from build123d import *

# Parameters (mm, degrees)
BOSS_EXTRUDE1_DEPTH = 40.1
SKETCH3_R           = 1.35
CUT_EXTRUDE2_DEPTH  = 50.8
SKETCH4_R           = 1.016
CUT_EXTRUDE3_DEPTH  = 50.8
SKETCH6_W           = 62.086073973
SKETCH6_H           = 34.1
CUT_EXTRUDE4_DEPTH  = 6
BOSS_EXTRUDE5_DEPTH = 2
FILLET1_R           = 1
CUT_EXTRUDE5_DEPTH  = 101.73954578


with BuildPart() as part:
    # Sketch1 → Boss-Extrude1 (new body)
    with BuildSketch(Plane.XY):
        Polygon((0, 0), (0, 52.578), (6, 52.578), (6, 8.5), (76, 8.5), (76, 0), align=None)
    extrude(amount=BOSS_EXTRUDE1_DEPTH)

    # Sketch3 → Cut-Extrude2 (cut)
    with BuildSketch(Plane.XY.offset(40.1)):
        with Locations((27.996, 2.8)):
            Circle(SKETCH3_R)
        with Locations((49.996, 2.8)):
            Circle(SKETCH3_R)
        with Locations((71.996, 2.8)):
            Circle(SKETCH3_R)
    extrude(amount=-CUT_EXTRUDE2_DEPTH, mode=Mode.SUBTRACT)

    # Sketch4 → Cut-Extrude3 (cut)
    with BuildSketch(Plane.ZY):
        with Locations((27.88, 17.6)):
            Circle(SKETCH4_R)
        with Locations(Location((11.88, 17.6, 0), (0, 0, 270))):
            Circle(SKETCH4_R)
        with Locations((27.88, 49.6)):
            Circle(SKETCH4_R)
        with Locations(Location((11.88, 49.6, 0), (0, 0, 270))):
            Circle(SKETCH4_R)
    extrude(amount=-CUT_EXTRUDE3_DEPTH, mode=Mode.SUBTRACT)

    # Sketch6 → Cut-Extrude4 (cut)
    with BuildSketch(Plane.XZ):
        with Locations((50.043036987, 20.05)):
            Rectangle(SKETCH6_W, SKETCH6_H)
    extrude(amount=-CUT_EXTRUDE4_DEPTH, mode=Mode.SUBTRACT)

    # Sketch16 → Boss-Extrude5 (add)
    with BuildSketch(Plane.XY.offset(40.1)):
        Polygon((6, 8.5), (26, 8.5), (6, 33.5), align=None)
    boss_extrude5 = extrude(amount=-BOSS_EXTRUDE5_DEPTH)

    # Mirror2: Boss-Extrude5 across plane
    add(boss_extrude5.mirror(Plane(origin=(0, 0, 20.05), x_dir=(1, 0, 0), z_dir=(0, 0, -1))))

    # Fillet1
    fillet1_edges = [part.edges().sort_by_distance(p)[0] for p in [
        (0, 0, 20.05),
        (76, 0, 38.6),
        (3, 52.578, 40.1),
        (76, 0, 1.5),
        (3, 52.578, 0),
    ]]
    fillet(fillet1_edges, radius=FILLET1_R)

    # Sketch17 → Cut-Extrude5 (cut, through all)
    with BuildSketch(Plane.XY.offset(40.1)):
        with BuildLine():
            Line((17.4625, 0), (17.4625, 8.5))
            Line((17.4625, 8.5), (6, 19.9625))
            Line((6, 19.9625), (6, 33.5))
            Line((6, 33.5), (26, 8.5))
            Line((26, 8.5), (76, 8.5))
            Line((76, 8.5), (76, 1))
            ThreePointArc((76, 1), (75.707106781, 0.292893219), (75, 0))
            Line((75, 0), (17.4625, 0))
        make_face()
    extrude(amount=-CUT_EXTRUDE5_DEPTH, mode=Mode.SUBTRACT)


solid = part.part
The listing builds one solid part. Answer for the finished solid, in the listing's coordinates (mm). A direction names the side the tool comes from. Coordinates: 2 decimals unless noted, no trailing zeros. Loops run counter-clockwise (first coordinate to the right, second up) from the corner with the lowest first, then second, coordinate; pieces in that order, holes last. Notation, with made-up numbers: (-23.75, -4.75) -> (3.25, -4.75) arc R17 ccw to (3.25, 26.25) -> close; hole circle Ø1 at (49, 67). An arc over 180 degrees is marked (long way). Answer in a Markdown table with one row per item. Add a question column.
1. Determine the mould class of faces 1 (the cylindrical face through (2.96, 48.7, 28.35)), 2 (the flat face through (3, 52.578, 20)), 3 (the cylindrical face through (2.958, 18.406, 11.262)), 4 (the flat face through (17.462, 4, 20)) for opening direction Y: +Y half, -Y half, draft (parallel to the pull), parting line (faces both ways), or undercut.
2. The part is cut by section C-C, the plane z = 27.88. Write down the section's boundary in (x, y), then the cut area to 3 significant figures.
3. The part is cut by section D-D, the plane x = 10. Write down the section's boundary in (y, z), then the cut area to 3 significant figures.
4. The part is cut by section A-A, the plane y = 49.6. Write down the section's boundary in (x, z), then the cut area to 3 significant figures.
5. For faces 5 (the flat face through (9, 12, 2)), 6 (the flat face through (5, 20, 0)), determine the directions among +Z, -Z, +X, -X, +Y, -Y from which every point of the face is accessible in a straight line to the end or side of a thin tool.
6. The part is cut by section B-B, the plane z = 23.5. Write down the section's boundary in (x, y), then the cut area to 3 significant figures.
7. Consider line 1 (Y direction, x = 4.8, z = 27.88); line 2 (Y direction, x = 16.25, z = 36); line 3 (X direction, y = 14.5, z = 31). Determine where each line is inside the solid, lowest interval first. Write a range as [from, to].
8. Flat-ended cylindrical pins translate along their axes: P1, Ø9, axis at x = 13, z = 12.5, coming from the +Y side; P2, Ø20, axis at y = 31, z = 28.5, coming from the +X side; P3, Ø1.6, axis at y = 49.6, z = 27.88, coming from the -X side. Find the tip coordinate at first contact, or state that the pin passes through.
Answer below:
| question | item | result |
|---|---|---|
| 1 | face 1 | undercut |
| 1 | face 2 | +Y half |
| 1 | face 3 | undercut |
| 1 | face 4 | draft |
| 2 | outline | (0, 1) arc R1 ccw to (1, 0) -> (17.46, 0) -> (17.46, 8.5) -> (6, 8.5) -> (6, 16.58) -> (0, 16.58) -> close; (0, 18.62) -> (6, 18.62) -> (6, 48.58) -> (0, 48.58) -> close; (0, 50.62) -> (6, 50.62) -> (6, 52.58) -> (0, 52.58) -> close |
| 2 | area | 388 mm2 |
| 3 | outline | (0, 0) -> (15.96, 0) -> (15.96, 2) -> (8.5, 2) -> (8.5, 38.1) -> (15.96, 38.1) -> (15.96, 40.1) -> (0, 40.1) -> close |
| 3 | area | 371 mm2 |
| 4 | outline | (0, 0) -> (6, 0) -> (6, 10.86) -> (0, 10.86) -> close; (0, 12.9) -> (6, 12.9) -> (6, 26.86) -> (0, 26.86) -> close; (0, 28.9) -> (6, 28.9) -> (6, 40.1) -> (0, 40.1) -> close |
| 4 | area | 216 mm2 |
| 5 | face 5 | +X, +Y |
| 5 | face 6 | -Z, +X, -X, +Y, -Y |
| 6 | outline | (0, 1) arc R1 ccw to (1, 0) -> (17.46, 0) -> (17.46, 8.5) -> (6, 8.5) -> (6, 52.58) -> (0, 52.58) -> close |
| 6 | area | 413 mm2 |
| 7 | line 1 | [0, 16.58], [18.62, 48.58], [50.62, 52.58] |
| 7 | line 2 | [0, 8.5] |
| 7 | line 3 | [0, 6] |
| 8 | P1 | y = 8.5 |
| 8 | P2 | x = 6 |
| 8 | P3 | through |
